```python
from build123d import *

# Parameters (mm, degrees)
F0_W     = 20
F0_H     = 20
F1_DEPTH = 20
F2_R     = 5
F3_DEPTH = 25
F4_R     = 30
F5_DEPTH = 5
F6_SIZE  = 1.5
F7_T     = -1


with BuildPart() as f1:
    # F0 (on Top) → F1 (new body)
    with BuildSketch(Plane.XY):
        Rectangle(F0_W, F0_H)
    extrude(amount=F1_DEPTH)

    # F2 (on face) → F3 (cut)
    with BuildSketch(Plane.XY.offset(20)):
        Circle(F2_R)
    extrude(amount=-F3_DEPTH, mode=Mode.SUBTRACT)

    # F4 (on face) → F5 (join)
    with BuildSketch(Plane.XY.offset(20)):
        Circle(F4_R)
    extrude(amount=F5_DEPTH)

    # F6
    f6_edges = [f1.edges().sort_by_distance(p)[0] for p in [
        (10, 0, 0),
        (0, 10, 0),
        (-10, 0, 0),
        (0, -10, 0),
    ]]
    chamfer(f6_edges, length=F6_SIZE)

    # F7
    f7_openings = [f1.faces().sort_by_distance(p)[0] for p in [
        (0, 0, 25),
    ]]
    offset(amount=F7_T, openings=f7_openings, kind=Kind.INTERSECTION)


solid = f1.part
```
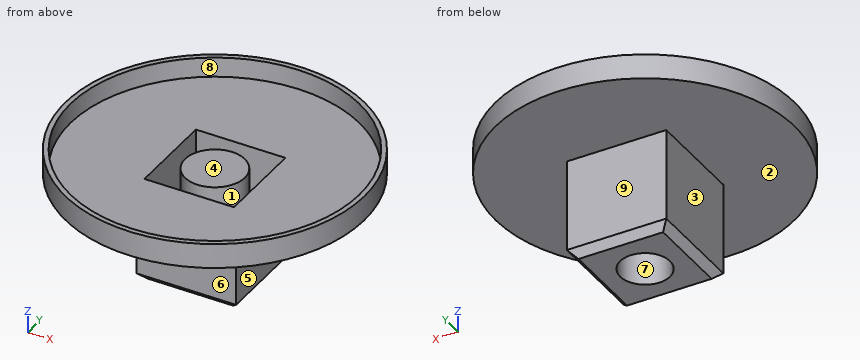
Input: part model. Units: mm. Frame: model coordinates. Face numbers are marked on the shaded views. A direction names the side the tool comes from. Coordinates: 2 decimals unless noted, no trailing zeros. Loops run counter-clockwise (first coordinate to the right, second up) from the corner with the lowest first, then second, coordinate; pieces in that order, holes last.
Q1. Section B-B, the plane x = 0. Return the cut outline in (y, z).
Results are:
outline: (-30, 20) - (-10, 20) - (-10, 1.5) - (-8.5, 0) - (-5, 0) - (-5, 20) - (5, 20) - (5, 0) - (8.5, 0) - (10, 1.5) - (10, 20) - (30, 20) - (30, 25) - (29, 25) - (29, 21) - (9, 21) - (9, 1.91) - (8.09, 1) - (6, 1) - (6, 21) - (-6, 21) - (-6, 1) - (-8.09, 1) - (-9, 1.91) - (-9, 21) - (-29, 21) - (-29, 25) - (-30, 25) - close
Q2. Contact query for flat-ended pins moving along their axis: pin 1 (3.5 mm diameter, centred on x = -1.5, y = 3, fed in from +Z); pin 2 (5.5 mm diameter, centred on y = 0, z = 10, fed in from -X); pin 3 (11 mm diameter, centred on x = 0.5, y = -2, fed in from -Z); pin 4 (5 mm diameter, centred on y = 12.5, z = 21.5, fed in from -X). Output: stop coordinate, or through.
Results are:
pin 1: stops at z = 21
pin 2: stops at x = -10
pin 3: stops at z = 0
pin 4: stops at x = -28.28
Q3. Section D-D, the plane z = 23.25. Return the cut outline in (x, y), and give its area (3 significant figures).
Results are:
outline: circle Ø60 at (0, 0); hole circle Ø58 at (0, 0)
area: 185 mm2
Q4. Mould query, pull axis X, two halves, no side actions, for the marked faces 1, 2, 3 and 4. Classes: +X half, -X half, draft (parallel to the pull), parting line (faces both ways), or undercut.
Results are:
face 1: undercut
face 2: draft
face 3: -X half
face 4: undercut
Q5. Set-up query: the marked faces 5, 6, 7, 8 and 9. Return all of +Z, -Z, +X, -X, +Y, -Y with unobstructed straight access to the full face (end or side cutting, diameter ignored); none if empty.
Results are:
face 5: -Z, +X, +Y, -Y
face 6: -Z, +X, -X, -Y
face 7: -Z
face 8: +Z
face 9: -Z, +X, -X, +Y
Q6. Section C-C, the plane y = 16.5. Return the cut outline in (x, z).
Results are:
outline: (-25.05, 20) - (25.05, 20) - (25.05, 25) - (23.85, 25) - (23.85, 21) - (-23.85, 21) - (-23.85, 25) - (-25.05, 25) - close
Q7. Section A-A, the plane z = 4. Return the cut outline in (x, y), and give its area (3 significant figures).
Results are:
outline: (-10, -10) - (10, -10) - (10, 10) - (-10, 10) - close; circle Ø12 at (0, 0); hole (-9, -9) - (9, -9) - (9, 9) - (-9, 9) - close; hole circle Ø10 at (0, 0)
area: 111 mm2
Q8. Line query: line 1 along Y through (x, z) = (0, 12.5); line 2 along Y through (x, z) = (0, 22.5); line 3 along X through (y, z) = (7.5, 16). Output: solid intervals per line, ascending.
Results are:
line 1: y = -10 to -9, -6 to -5, 5 to 6, 9 to 10
line 2: y = -30 to -29, 29 to 30
line 3: x = -10 to -9, 9 to 10
